Design review of the part built by this model. Coordinates are the model's own, in mm. Face numbers are marked on the shaded views. A direction names the side the tool comes from. Coordinates: 2 decimals unless noted, no trailing zeros. Write each loop counter-clockwise with the first axis right and the second up, starting at its lowest first coordinate (ties: lowest second). Pieces come first, ordered by that corner, then holes.
Q1. Add section B-B, the plane z = -1.1. Give the boundary of the cut face in (x, y).
Q2. Add section C-C, the plane y = 30.48. Give the number of separate pieces and of enclosed holes in the cut face, plus the area to 3 significant figures.
Q3. Clearance check with flat-ended pins moving along their axes: pin 1 Ø6 at (y, z) = (30.48, -1.1) entering from -X; pin 2 Ø8 at (x, z) = (-36.5, -11) entering from +Y. State where each tip first meets the part, or that it passes through.
Q4. To check wall thickness, follow probe 1 along Z at (x, y) = (-66.25, 30.48); probe 2 along X at (y, z) = (16, 7.5); probe 3 along Y at (x, z) = (-71.75, -1.1). State the ranges of each line that lie inside material, in increasing order.
Q5. The part is to be moulded in two halves that separate along X. For the marked faces 3, 4 and 5, say which applies: +X half, -X half, draft (parallel to the pull), parting line (faces both ways), or undercut.
Q6. Add section A-A, the plane y = 18. Give the boundary of the cut face in (x, z), plus the area to 3 significant figures.
Q7. Add section D-D, the plane z = 20.5. Give the boundary of the cut face in (x, y), plus the area to 3 significant figures.
Q8. Machinability: for the marked faces 1 and 2, which of the approach directions +Z, -Z, +X, -X, +Y, -Y give a long, thin tool a straight path to every point of the face, cutting with its end or side? Answer none if there is none.
Autodesk Inventor part; units mm, degrees
ref_plane "YZ Plane" through (0, 0, 0) normal (1, 0, 0) x (0, 1, 0)
ref_plane "XZ Plane" through (0, 0, 0) normal (0, 1, 0) x (-1, 0, 0)
ref_plane "XY Plane" through (0, 0, 0) normal (0, 0, 1) x (1, 0, 0)
sketch "Sketch2" plane through (0, 0, 0) normal (0, 1, 0) x (-1, 0, 0)
  line L0 (-76.2, -38.1) -> (76.2, -38.1)
  line L1 (76.2, -38.1) -> (76.2, 38.1)
  line L2 (76.2, 38.1) -> (-76.2, 38.1)
  line L3 (-76.2, 38.1) -> (-76.2, -38.1)
  line L4 (-76.2, -38.1) -> (76.2, 38.1) construction
  line L5 (76.2, -38.1) -> (-76.2, 38.1) construction
  point P0 (0, 0)
  dimension "d0" = 152.4
  dimension "d1" = 76.2
extrude "Extrusion1" add sketch "Sketch2" along normal blind 50.8
sketch "Sketch3" plane through (0, 50.8, 0) normal (0, 1, 0) x (1, 0, 0)
  line L0 (63.5, -38.1) -> (-63.5, -38.1)
  line L1 (-63.5, -38.1) -> (-63.5, 38.1)
  line L2 (-63.5, 38.1) -> (63.5, 38.1)
  line L3 (63.5, 38.1) -> (63.5, -38.1)
  line L4 (63.5, -38.1) -> (-63.5, 38.1) construction
  line L5 (-63.5, -38.1) -> (63.5, 38.1) construction
  point P0 (0, 0)
  dimension "d4" = 127
  dimension "d5" = 76.2
extrude "Extrusion2" cut sketch "Sketch3" against normal blind 38.1
sketch "Sketch4" plane through (63.5, 50.8, -38.1) normal (-1, 0, 0) x (0, 0, 1)
  line L0 (0, 0) -> (76.2, 0)
  line L1 (0, -38.1) -> (0, 0)
  point P0 (38.1, -50.8)
  point P1 (10.16, -20.32)
  dimension "d8" = 20.32
  dimension "d9" = 10.16
hole "Hole1" at (63.5, 30.48, -27.94) direction (1, 0, 0) diameter 10 end through all
sketch "Sketch5" plane through (63.5, 50.8, -38.1) normal (-1, 0, 0) x (0, 0, 1)
  line L0 (0, 0) -> (76.2, 0)
  line L1 (76.2, 0) -> (76.2, -38.1)
  point P0 (38.1, -50.8)
  point P1 (66.04, -20.32)
  dimension "d17" = 20.32
  dimension "d18" = 10.16
hole "Hole2" at (63.5, 30.48, 27.94) direction (1, 0, 0) diameter 10 end through all
sketch "Sketch6" plane through (-63.5, 50.8, 38.1) normal (1, 0, 0) x (0, 0, -1)
  line L0 (0, 0) -> (76.2, 0)
  line L1 (0, -38.1) -> (0, 0)
  line L2 (76.2, 0) -> (76.2, -38.1)
  point P0 (38.1, -50.8)
  point P1 (10.16, -20.32)
  point P2 (66.04, -20.32)
  dimension "d26" = 20.32
  dimension "d27" = 10.16
  dimension "d28" = 20.32
  dimension "d29" = 10.16
hole "Hole3" at (-63.5, 30.48, 27.94) at (-63.5, 30.48, -27.94) direction (-1, 0, 0) diameter 10 end through all
sketch "Sketch7" plane through (63.5, 50.8, -38.1) normal (-1, 0, 0) x (0, 0, 1)
  line L0 (0, 0) -> (76.2, 0)
  line L1 (0, -38.1) -> (0, 0)
  point P0 (38.1, -50.8)
  point P1 (37, -20.32)
  dimension "d37" = 20.32
  dimension "d38" = 37
hole "Hole4" at (63.5, 30.48, -1.1) direction (1, 0, 0) diameter 10 end through all
sketch "Sketch8" plane through (-76.2, 0, -38.1) normal (-1, 0, 0) x (0, 0, 1)
  line L0 (0, 50.8) -> (76.2, 50.8)
  line L1 (0, 0) -> (0, 50.8)
  point P0 (38.1, 0)
  point P1 (37, 30.48)
  dimension "d46" = 20.32
  dimension "d47" = 37
hole "Hole5" at (-76.2, 30.48, -1.1) direction (1, 0, 0) diameter 10 end through all
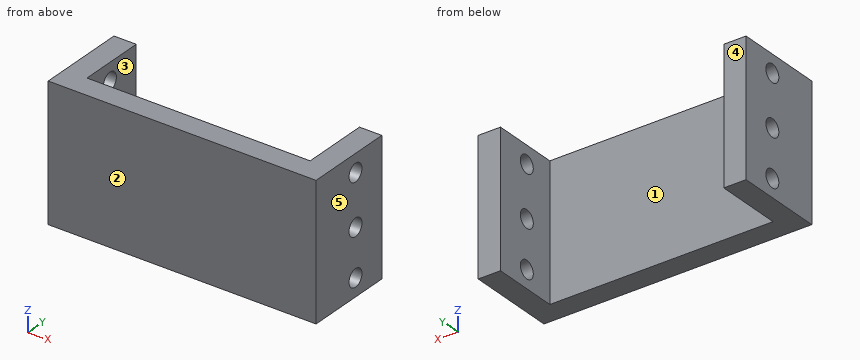
Here are the results:
1. outline: (-76.2, 0) - (76.2, 0) - (76.2, 25.48) - (63.5, 25.48) - (63.5, 12.7) - (-63.5, 12.7) - (-63.5, 25.48) - (-76.2, 25.48) - close; (-76.2, 35.48) - (-63.5, 35.48) - (-63.5, 50.8) - (-76.2, 50.8) - close; (63.5, 35.48) - (76.2, 35.48) - (76.2, 50.8) - (63.5, 50.8) - close
2. separate pieces: 8
2. enclosed holes: 0
2. area: 1,170 mm2
3. pin 1: passes through
3. pin 2: stops at y = 12.7
4. probe 1: z = -38.1 to -32.94, -22.94 to -6.1, 3.9 to 22.94, 32.94 to 38.1
4. probe 2: x = -76.2 to -63.5, 63.5 to 76.2
4. probe 3: y = 0 to 25.48, 35.48 to 50.8
5. face 3: undercut
5. face 4: draft
5. face 5: +X half
6. outline: (-76.2, -38.1) - (-63.5, -38.1) - (-63.5, 38.1) - (-76.2, 38.1) - close; (63.5, -38.1) - (76.2, -38.1) - (76.2, 38.1) - (63.5, 38.1) - close
6. area: 1,940 mm2
7. outline: (-76.2, 0) - (76.2, 0) - (76.2, 50.8) - (63.5, 50.8) - (63.5, 12.7) - (-63.5, 12.7) - (-63.5, 50.8) - (-76.2, 50.8) - close
7. area: 2,900 mm2
8. face 1: +Z, -Z, +Y
8. face 2: +Z, -Z, +X, -X, -Y
